Part model, mm, in its own coordinate system. Face numbers are marked on the shaded views. Coordinates: 2 decimals unless noted, no trailing zeros. Write each loop counter-clockwise with the first axis right and the second up, starting at its lowest first coordinate (ties: lowest second). Pieces come first, ordered by that corner, then holes. Notation, with made-up numbers: (-38, 62) -> (18, 62) arc R26 cw to (18, 99) -> close; hole circle Ø7 at (-34.75, 26). An arc over 180 degrees is marked (long way). Write item = value, one per line. Start each with the question number.
Q1. Band-saw the part on A-A, the plane x = -10. List the corners of the cut face in (y, z).
Q2. Band-saw the part on B-B, the plane z = 0. List the corners of the cut face in (x, y), plus the area to 3 significant figures.
Q3. Pin check, flat tips, straight feed: P1, Ø2.5, axis at x = -10, z = 0, coming from the -Y side; P2, Ø1.5, axis at y = 2.5, z = -14.5, coming from the +X side; P3, Ø2, axis at x = 33, y = 2.5, coming from the -Z side; P4, Ø1, axis at y = 4.5, z = 5, coming from the -X side. Stop position of each tip, or through.
Q4. Probe line 1 (X direction, y = 3.25, z = 0); line 2 (X direction, y = 2.6, z = 14); line 3 (X direction, y = 3.9, z = 6.75). List the from-to ranges inside material, lowest first.
Q5. Pull direction X, two halves, no side cores. Call the marked faces 1, 2 and 3: released by +X, released by -X, zero draft, split by the parting line, or undercut.
Q6. Band-saw the part on C-C, the plane y = 3.9. Give the number of separate pieces and of enclosed holes in the cut face, plus the area to 3 significant figures.
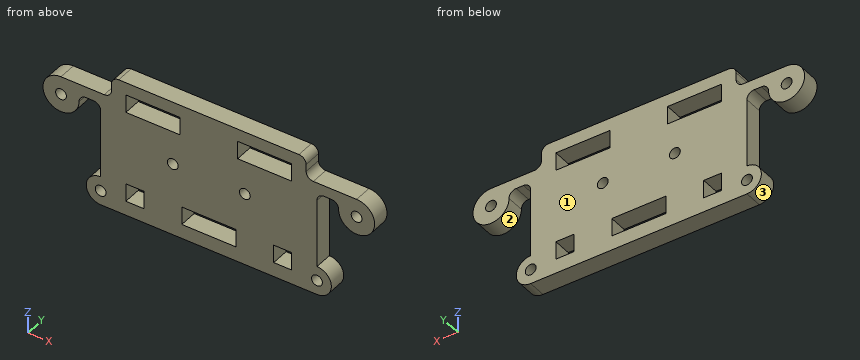
from build123d import *

# Parameters (mm, degrees)
SKETCH1_R           = 1.5
SKETCH1_W           = 5
SKETCH1_H           = 5
SKETCH1_W_2         = 15
BOSS_EXTRUDE1_DEPTH = 5


with BuildPart() as part:
    # Sketch1 → Boss-Extrude1 (new body)
    with BuildSketch(Plane(origin=(0, 0, 0), x_dir=(1, 0, 0), z_dir=(0, 1, 0))):
        with BuildLine():
            Line((-29, -11.75), (-30, -11.75))
            Line((-30, -11.75), (-41, -11.75))
            ThreePointArc((-41, -11.75), (-44.535533906, -3.214466094), (-36, -6.75))
            ThreePointArc((-36, -6.75), (-35.414213562, -8.164213562), (-34, -8.75))
            Line((-34, -8.75), (-32, -8.75))
            ThreePointArc((-32, -8.75), (-30.585786438, -8.164213562), (-30, -6.75))
            Line((-30, -6.75), (-30, 12.25))
            ThreePointArc((-30, 12.25), (-34, 16.25), (-30, 20.25))
            Line((-30, 20.25), (30, 20.25))
            ThreePointArc((30, 20.25), (34, 16.25), (30, 12.25))
            Line((30, 12.25), (30, -6.75))
            ThreePointArc((30, -6.75), (30.585786438, -8.164213562), (32, -8.75))
            Line((32, -8.75), (34, -8.75))
            ThreePointArc((34, -8.75), (35.414213562, -8.164213562), (36, -6.75))
            ThreePointArc((36, -6.75), (44.535533906, -3.214466094), (41, -11.75))
            Line((41, -11.75), (30, -11.75))
            Line((30, -11.75), (29, -11.75))
            ThreePointArc((29, -11.75), (27.585786438, -12.335786438), (27, -13.75))
            Line((27, -13.75), (27, -15.75))
            ThreePointArc((27, -15.75), (26.414213562, -17.164213562), (25, -17.75))
            Line((25, -17.75), (-25, -17.75))
            ThreePointArc((-25, -17.75), (-26.414213562, -17.164213562), (-27, -15.75))
            Line((-27, -15.75), (-27, -13.75))
            ThreePointArc((-27, -13.75), (-27.585786438, -12.335786438), (-29, -11.75))
        make_face()
        with Locations((-10, 0)):
            Circle(SKETCH1_R, mode=Mode.SUBTRACT)
        with Locations((10, 0)):
            Circle(SKETCH1_R, mode=Mode.SUBTRACT)
        with Locations((-30, 16.25)):
            Circle(SKETCH1_R, mode=Mode.SUBTRACT)
        with Locations((30, 16.25)):
            Circle(SKETCH1_R, mode=Mode.SUBTRACT)
        with Locations((41, -6.75)):
            Circle(SKETCH1_R, mode=Mode.SUBTRACT)
        with Locations((-41, -6.75)):
            Circle(SKETCH1_R, mode=Mode.SUBTRACT)
        with Locations((-20.5, 13.75)):
            Rectangle(SKETCH1_W, SKETCH1_H, mode=Mode.SUBTRACT)
        with Locations((0, 13.75)):
            Rectangle(SKETCH1_W_2, SKETCH1_H, mode=Mode.SUBTRACT)
        with Locations((20.5, 13.75)):
            Rectangle(SKETCH1_W, SKETCH1_H, mode=Mode.SUBTRACT)
        with Locations((-15.5, -11.75)):
            Rectangle(SKETCH1_W_2, SKETCH1_H, mode=Mode.SUBTRACT)
        with Locations((15.5, -11.75)):
            Rectangle(SKETCH1_W_2, SKETCH1_H, mode=Mode.SUBTRACT)
    extrude(amount=BOSS_EXTRUDE1_DEPTH)


solid = part.part
Ans:
q1.outline = (0, -20.25) -> (5, -20.25) -> (5, -1.5) -> (0, -1.5) -> close; (0, 1.5) -> (5, 1.5) -> (5, 9.25) -> (0, 9.25) -> close; (0, 14.25) -> (5, 14.25) -> (5, 17.75) -> (0, 17.75) -> close
q2.outline = (-30, 0) -> (-11.5, 0) -> (-11.5, 5) -> (-30, 5) -> close; (-8.5, 0) -> (8.5, 0) -> (8.5, 5) -> (-8.5, 5) -> close; (11.5, 0) -> (30, 0) -> (30, 5) -> (11.5, 5) -> close
q2.area = 270 mm2
q3.P1 = through
q3.P2 = 33.87
q3.P3 = -19.71
q3.P4 = -45.84
q4.line_1 = -30 to -11.5, -8.5 to 8.5, 11.5 to 30
q4.line_2 = -27 to -23, -8 to 8, 23 to 27
q4.line_3 = -46 to -42.5, -39.5 to -36, -30 to 30, 36 to 39.5, 42.5 to 46
q5.face_1 = zero draft
q5.face_2 = undercut
q5.face_3 = released by -X
q6.separate_pieces = 1
q6.enclosed_holes = 11
q6.area = 2,180 mm2
